from build123d import *

# Parameters (mm, degrees)
SKETCH_1_R          = 28.5
EXTRUDE_1_DEPTH     = 45
SKETCH_2_R          = 17.5
CUT_EXTRUDE_1_DEPTH = 30
SKETCH_3_R          = 1.5
CUT_EXTRUDE_2_DEPTH = 6
SKETCH_7_W          = 5
SKETCH_7_H          = 14
CUT_EXTRUDE_3_DEPTH = 45
SKETCH_8_W          = 7
SKETCH_8_H          = 9
CUT_EXTRUDE_4_DEPTH = 90
SKETCH_9_R          = 1.5
CUT_EXTRUDE_5_DEPTH = 10


with BuildPart() as part:
    # Sketch 1 → Extrude 1 (new body)
    with BuildSketch(Plane(origin=(0, 0, 0), x_dir=(1, 0, 0), z_dir=(0, 1, 0))):
        Circle(SKETCH_1_R)
    extrude(amount=EXTRUDE_1_DEPTH)

    # Sketch 2 → Cut-Extrude 1 (cut)
    with BuildSketch(Plane(origin=(0, 45, 0), x_dir=(1, 0, 0), z_dir=(0, 1, 0))):
        Circle(SKETCH_2_R)
    extrude(amount=-CUT_EXTRUDE_1_DEPTH, mode=Mode.SUBTRACT)

    # Sketch 3 → Cut-Extrude 2 (cut)
    with BuildSketch(Plane.XZ):
        with Locations((-19, 0)):
            Circle(SKETCH_3_R)
        with Locations((0, 19)):
            Circle(SKETCH_3_R)
        with Locations((19, 0)):
            Circle(SKETCH_3_R)
        with Locations((0, -19)):
            Circle(SKETCH_3_R)
    extrude(amount=-CUT_EXTRUDE_2_DEPTH, mode=Mode.SUBTRACT)

    # Sketch 7 → Cut-Extrude 3 (cut, symmetric)
    with BuildSketch(Plane(origin=(0, 0, 0), x_dir=(0, 1, 0), z_dir=(0.707106781, 0, -0.707106781))):
        with Locations((4, 0)):
            Rectangle(SKETCH_7_W, SKETCH_7_H)
    extrude(amount=CUT_EXTRUDE_3_DEPTH, both=True, mode=Mode.SUBTRACT)

    # Sketch 8 → Cut-Extrude 4 (cut)
    with BuildSketch(Plane(origin=(0, 0, 0), x_dir=(0, 1, 0), z_dir=(0.707106781, 0, 0.707106781))):
        with Locations((5, 0)):
            Rectangle(SKETCH_8_W, SKETCH_8_H)
    extrude(amount=-CUT_EXTRUDE_4_DEPTH, mode=Mode.SUBTRACT)

    # Sketch 9 → Cut-Extrude 5 (cut)
    with BuildSketch(Plane(origin=(0, 45, 0), x_dir=(1, 0, 0), z_dir=(0, 1, 0))):
        with Locations((-25, 0)):
            Circle(SKETCH_9_R)
        with Locations((-12.5, 21.650635095)):
            Circle(SKETCH_9_R)
        with Locations((12.5, 21.650635095)):
            Circle(SKETCH_9_R)
        with Locations((25, 0)):
            Circle(SKETCH_9_R)
        with Locations((12.5, -21.650635095)):
            Circle(SKETCH_9_R)
        with Locations((-12.5, -21.650635095)):
            Circle(SKETCH_9_R)
    extrude(amount=-CUT_EXTRUDE_5_DEPTH, mode=Mode.SUBTRACT)


solid = part.part
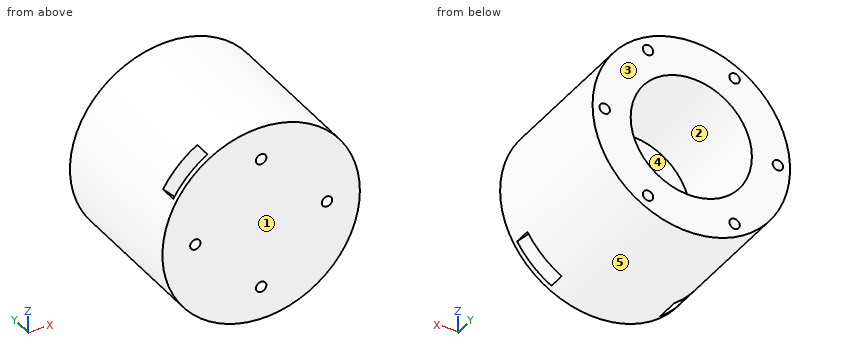
Geometry: final body of the model. Coordinates: model frame, mm. Face numbers are marked on the shaded views. A direction names the side the tool comes from. Coordinates: 2 decimals unless noted, no trailing zeros. Order: outer loops, then holes, each group sorted by start corner. A loop starts at its lowest first (then second) coordinate and runs counter-clockwise, first axis right, second up.
(1) First-contact query: pin 1 (1.5 mm diameter, centred on x = 1.5, y = 7.5, fed in from -Z); pin 2 (1.5 mm diameter, centred on x = 12.5, z = 22, fed in from +Y); pin 3 (1 mm diameter, centred on x = 1.5, z = -4, fed in from +Y). Flat tips, straight axial feed; report the tip coordinate or a pass-through.
(2) Section query B-B (z = 11.5). Return the cut outline in (x, y), plus the area to 3 significant figures.
(3) Section query C-C (x = -19.5). Return the cut outline in (y, z), plus the area to 3 significant figures.
(4) Access query for the marked faces 1 and 2. Directions: +Z, -Z, +X, -X, +Y, -Y. A direction counts if a zero-diameter tool reaches every point of the face in a straight line with its end or side. Return the directions, or none.
(5) Draft query along Z for the marked faces 3, 4 and 5. Return one class per face: pulls with the +Z half, pulls with the -Z half, needs draft (parallel to the pull), parting line crosses it, or undercut.
(6) Section query D-D (y = 25). Return the cut outline in (x, z).
(7) Material intervals for probe 1 along X at (y, z) = (39.5, 0); probe 2 along Y at (x, z) = (-3, 9.5); probe 3 along Y at (x, z) = (-18.5, 10.5), sorted ascending.
(8) Section query A-A (x = -13). Return the cut outline in (y, z).
Solution:
1. pin 1: stops at z = -28.49
1. pin 2: stops at y = 35
1. pin 3: stops at y = 15
2. outline: (-26.08, 0) - (26.08, 0) - (26.08, 45) - (13.19, 45) - (13.19, 15) - (-13.19, 15) - (-13.19, 45) - (-26.08, 45) - close; hole (-21.4, 1.5) - (-1.6, 1.5) - (-1.6, 6.5) - (-21.4, 6.5) - close
2. area: 1,460 mm2
3. outline: (0, -20.78) - (1.5, -20.78) - (1.5, -13.14) - (8.5, -13.14) - (8.5, -20.78) - (45, -20.78) - (45, 20.78) - (6.5, 20.78) - (6.5, 9.6) - (1.5, 9.6) - (1.5, 20.78) - (0, 20.78) - (0, 1.41) - (6, 1.41) - (6, -1.41) - (0, -1.41) - close
3. area: 1,740 mm2
4. face 1: +Z, -Z, +X, -X, -Y
4. face 2: +Y
5. face 3: needs draft
5. face 4: undercut
5. face 5: parting line crosses it
6. outline: circle Ø57 at (0, 0); hole circle Ø35 at (0, 0)
7. probe 1: x = -28.5 to -26.5, -23.5 to -17.5, 17.5 to 23.5, 26.5 to 28.5
7. probe 2: y = 0 to 1.5, 6.5 to 15
7. probe 3: y = 0 to 1.5, 6.5 to 45
8. outline: (0, -25.36) - (45, -25.36) - (45, -23.06) - (35, -23.06) - (35, -20.24) - (45, -20.24) - (45, -11.72) - (15, -11.72) - (15, 11.72) - (45, 11.72) - (45, 20.24) - (35, 20.24) - (35, 23.06) - (45, 23.06) - (45, 25.36) - (0, 25.36) - close; hole (1.5, -19.36) - (8.5, -19.36) - (8.5, -6.64) - (1.5, -6.64) - close; hole (1.5, 3.1) - (6.5, 3.1) - (6.5, 22.9) - (1.5, 22.9) - close
